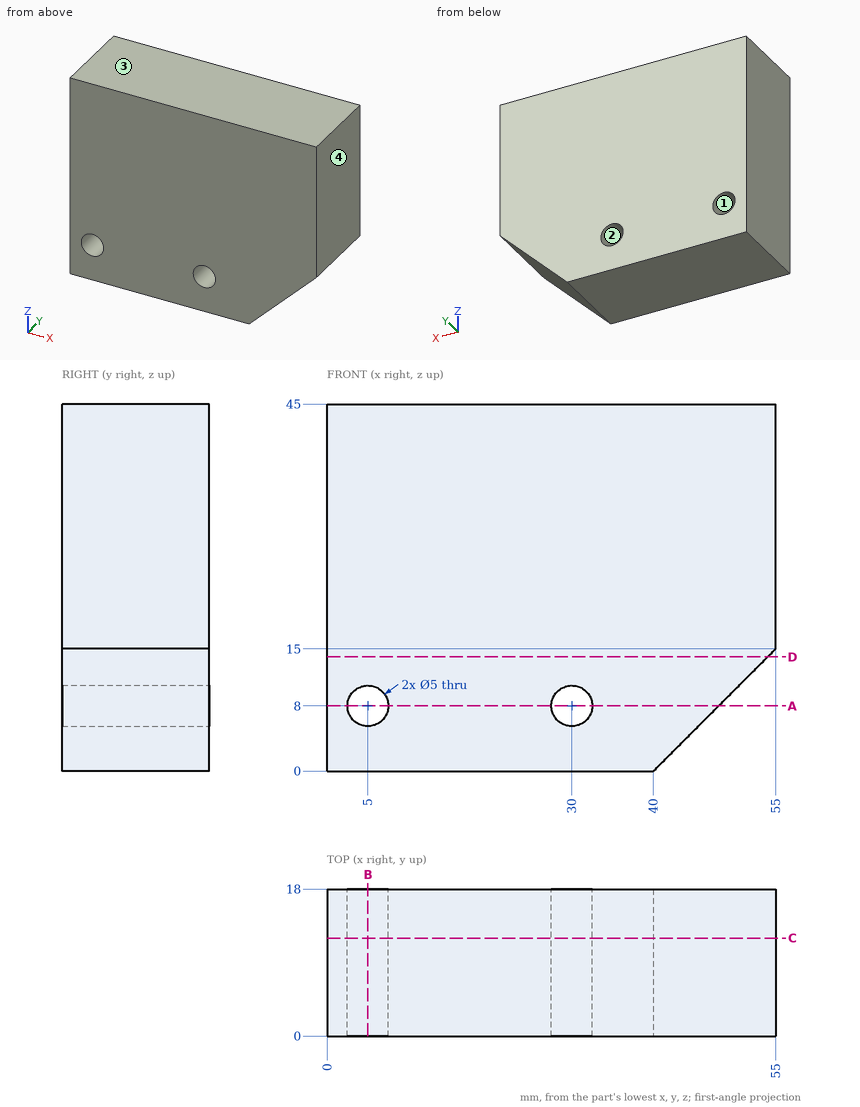
For this review, use the dimensioned drawing (mm, ordinates from the lowest corner) and the shaded views. Round coordinates to 2 decimals unless told otherwise and drop trailing zeros. Order: outer loops, then holes, each group sorted by start corner. A loop starts at its lowest first (then second) coordinate and runs counter-clockwise, first axis right, second up. Notation, with made-up numbers: M 77.25,-22 L 110.25,-22 A13 cw 110.25,-3 Z; hole C 33,-29.75 d8. An arc over 180 degrees is marked long. Use a Markdown table: item, result. Add a question column.
Item 1: Mouldability with a two-part tool opening along X and no side actions: class the marked faces 1, 2, 3 and 4 as released by +X, released by -X, zero draft, split by the parting line, or undercut.
Item 2: Add section A-A, the plane z = 8. Give the boundary of the cut face in (x, y).
Item 3: Insertion check: pin 1 (2 mm diameter, centred on x = 47, y = 9, fed in from -Z). The pin has a flat end and moves straight along its axis. Give the tip position at first contact, or say it passes through.
Item 4: Add section D-D, the plane z = 14. Give the boundary of the cut face in (x, y), then the cut area to 3 significant figures.
Item 5: To check wall thickness, follow line 1 along Z through (x, y) = (5, 5.75); line 2 along X through (y, z) = (3, 7); line 3 along Z through (x, y) = (6, 15.25). State the ranges of each line that lie inside material, in increasing order.
Item 6: Add section C-C, the plane y = 12. Give the boundary of the cut face in (x, z), then the cut area to 3 significant figures.
Item 7: Add section B-B, the plane x = 5. Give the boundary of the cut face in (y, z), then the cut area to 3 significant figures.
Geometry results:
| question | item | result |
|---|---|---|
| 1 | face 1 | undercut |
| 1 | face 2 | undercut |
| 1 | face 3 | zero draft |
| 1 | face 4 | released by +X |
| 2 | outline | M 0,0 L 2.5,0 L 2.5,18 L 0,18 Z; M 7.5,0 L 27.5,0 L 27.5,18 L 7.5,18 Z; M 32.5,0 L 48,0 L 48,18 L 32.5,18 Z |
| 3 | pin 1 | stops at z = 6 |
| 4 | outline | M 0,0 L 54,0 L 54,18 L 0,18 Z |
| 4 | area | 972 mm² |
| 5 | line 1 | z = 0 to 5.5, 10.5 to 45 |
| 5 | line 2 | x = 0 to 2.71, 7.29 to 27.71, 32.29 to 47 |
| 5 | line 3 | z = 0 to 5.71, 10.29 to 45 |
| 6 | outline | M 0,0 L 40,0 L 55,15 L 55,45 L 0,45 Z; hole C 5,8 d5; hole C 30,8 d5 |
| 6 | area | 2,320 mm² |
| 7 | outline | M 0,0 L 18,0 L 18,5.5 L 0,5.5 Z; M 0,10.5 L 18,10.5 L 18,45 L 0,45 Z |
| 7 | area | 720 mm² |
